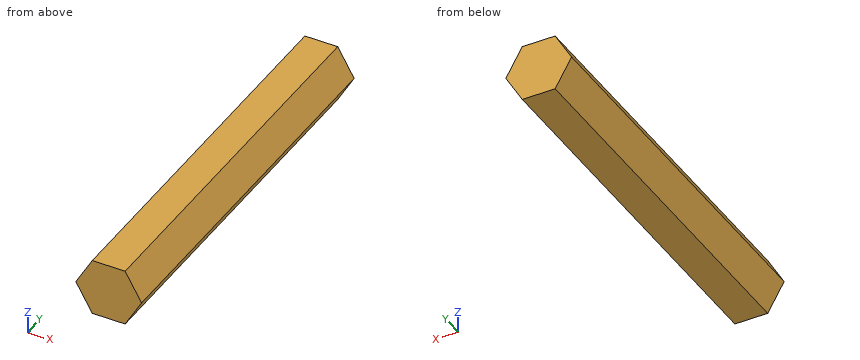
from build123d import *

# Parameters (mm, degrees)
F1_DEPTH = 28
F4_DEPTH = 28


with BuildPart() as f1:
    # F0 (on Front) → F1 (new body)
    with BuildSketch(Plane.XZ):
        Polygon((6.646589714, 11.5122310817), (-6.646589714, 11.5122310817), (-13.293179428, 0), (-6.646589714, -11.5122310817), (6.646589714, -11.5122310817), (13.293179428, 0), align=None)
    extrude(amount=F1_DEPTH)


with BuildPart() as f4:
    # F3 (on Front) → F4 (new body)
    with BuildSketch(Plane.XZ):
        Polygon((1.2, 2.0784609691), (-1.2, 2.0784609691), (-2.4, 0), (-1.2, -2.0784609691), (1.2, -2.0784609691), (2.4, 0), align=None)
    extrude(amount=F4_DEPTH)


solid = f4.part
Design review of the part built by this model. Coordinates are the model's own, in mm. Coordinates: 2 decimals unless noted, no trailing zeros. Order: outer loops, then holes, each group sorted by start corner. A loop starts at its lowest first (then second) coordinate and runs counter-clockwise, first axis right, second up. Notation, with made-up numbers: (1.5, 38) -> (40.5, 38) arc R10 cw to (40.5, 55) -> close; hole circle Ø3 at (-14, 64). An arc over 180 degrees is marked (long way). Use one line per item in the form item = value. Start each with the question number.
(1) Add section A-A on y = -16.75. State the section outline as (x, z) points.
(2) Add section B-B on x = 1.55. State the section outline as (y, z) points.
(3) Add section C-C on z = 0.4. State the section outline as (x, y) points.
(4) For probe 1 along Z at (x, y) = (1.7, -25.75); probe 2 along X at (y, z) = (-19.25, 1.45); probe 3 along Z at (x, y) = (1.85, -17.75), list the stretches that pass through material, from the lowest coordinate up.
Answer block:
q1.outline = (-2.4, 0) -> (-1.2, -2.08) -> (1.2, -2.08) -> (2.4, 0) -> (1.2, 2.08) -> (-1.2, 2.08) -> close
q2.outline = (-28, -1.47) -> (0, -1.47) -> (0, 1.47) -> (-28, 1.47) -> close
q3.outline = (-2.17, -28) -> (2.17, -28) -> (2.17, 0) -> (-2.17, 0) -> close
q4.probe_1 = -1.21 to 1.21
q4.probe_2 = -1.56 to 1.56
q4.probe_3 = -0.95 to 0.95
